from build123d import *

# Parameters (mm, degrees)
SKETCH1_R           = 2.5
BOSS_EXTRUDE1_DEPTH = 4.5


with BuildPart() as part:
    # Sketch1 → Boss-Extrude1 (new body)
    with BuildSketch(Plane.XY):
        Polygon((-206.5, 269.5), (204.5, 269.5), (204.5, 244.5), (178.5, 244.5), (178.5, 202.5), (187.5, 202.5), (187.5, 160.5), (204.5, 160.5), (204.5, -160.5), (178.5, -160.5), (178.5, -202.5), (187.5, -202.5), (187.5, -244.5), (204.5, -244.5), (204.5, -269.5), (-206.5, -269.5), (-206.5, -244.5), (-206.5, -160.5), (-206.5, -66), (-180.5, -66), (-180.5, 66), (-206.5, 66), (-206.5, 160.5), (-206.5, 244.5), align=None)
        with Locations((136.5, -257.5)):
            Circle(SKETCH1_R, mode=Mode.SUBTRACT)
        with Locations(Location((-138.5, -257.5, 0), (0, 0, 180))):
            Circle(SKETCH1_R, mode=Mode.SUBTRACT)
        with Locations((-138.5, 257.5)):
            Circle(SKETCH1_R, mode=Mode.SUBTRACT)
        with Locations(Location((136.5, 257.5, 0), (0, 0, 180))):
            Circle(SKETCH1_R, mode=Mode.SUBTRACT)
        with Locations((-194.5, 107.5)):
            Circle(SKETCH1_R, mode=Mode.SUBTRACT)
        with Locations(Location((-194.5, -107.5, 0), (0, 0, 180))):
            Circle(SKETCH1_R, mode=Mode.SUBTRACT)
        with Locations(Location((192.5, 107.5, 0), (0, 0, 180))):
            Circle(SKETCH1_R, mode=Mode.SUBTRACT)
        with Locations((192.5, -107.5)):
            Circle(SKETCH1_R, mode=Mode.SUBTRACT)
    extrude(amount=BOSS_EXTRUDE1_DEPTH)


solid = part.part
Verification items for the finished model (mm, model axes). Give positions to 0.01 mm unless a question says otherwise; leave off trailing zeros. Write each loop counter-clockwise with the first axis right and the second up, starting at its lowest first coordinate (ties: lowest second). Pieces come first, ordered by that corner, then holes. Notation, with made-up numbers: (41.25, 75) -> (80.25, 75) arc R22 cw to (80.25, 109) -> close; hole circle Ø2 at (-3.5, -13.75). An arc over 180 degrees is marked (long way). Use CSV: the item, a comma, the result in double quotes.
(1) Sectioned sample at B-B (y = -25). Record the cut outline in (x, z).
Derived:
outline,"(-180.5, 0) -> (204.5, 0) -> (204.5, 4.5) -> (-180.5, 4.5) -> close"
(2) Sectioned sample at A-A (z = 2.55). Give the number of separate pieces and of enclosed holes in the cut face, plus the area to 3 significant figures.
Derived:
separate pieces,"1"
enclosed holes,"8"
area,"214,000 mm^2"
(3) Material ranges on L1, parallel to Y at x = -194.5, z = 1.6; L2, parallel to Y at x = 192.5, z = 1.25; L3, parallel to Y at x = 182.5, z = 4.35, recorded low to high.
Derived:
L1,"y = -269.5 to -110, -105 to -66, 66 to 105, 110 to 269.5"
L2,"y = -269.5 to -244.5, -160.5 to -110, -105 to 105, 110 to 160.5, 244.5 to 269.5"
L3,"y = -269.5 to -202.5, -160.5 to 202.5, 244.5 to 269.5"
(4) Go/stop test with flat-tipped pins: pin 1 (2 mm diameter, centred on y = -176.5, z = 1.5, fed in from +X); pin 2 (2 mm diameter, centred on y = 3.5, z = 1.5, fed in from -X); pin 3 (1.3 mm diameter, centred on y = 185.5, z = 2, fed in from +X). Record where each tip stops, or that it passes through.
Derived:
pin 1,"stops at x = 178.5"
pin 2,"stops at x = -180.5"
pin 3,"stops at x = 187.5"
(5) Sectioned sample at C-C (y = 180.5). Record the cut outline in (x, z).
Derived:
outline,"(-206.5, 0) -> (187.5, 0) -> (187.5, 4.5) -> (-206.5, 4.5) -> close"
